For this review, take the finished solid that the model builds, in its own axes (mm). Face numbers are marked on the shaded views. A direction names the side the tool comes from. Give positions to 0.01 mm unless a question says otherwise; leave off trailing zeros. Loops run counter-clockwise (first coordinate to the right, second up) from the corner with the lowest first, then second, coordinate; pieces in that order, holes last. Notation, with made-up numbers: (82.25, 28.5) - (104.25, 28.5) arc R12 ccw to (104.25, 41.5) - close; hole circle Ø2 at (87, -33). An arc over 180 degrees is marked (long way). Answer as CSV lines item,"result".
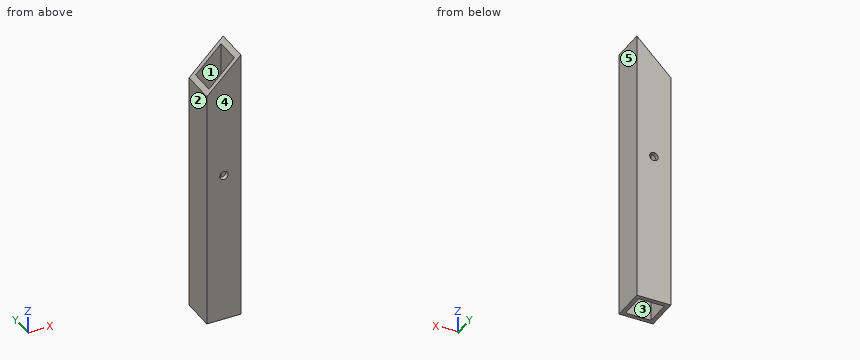
Autodesk Inventor part; units mm, degrees
ref_plane "YZ Plane" through (0, 0, 0) normal (1, 0, 0) x (0, 1, 0)
ref_plane "XZ Plane" through (0, 0, 0) normal (0, 1, 0) x (-1, 0, 0)
ref_plane "XY Plane" through (0, 0, 0) normal (0, 0, 1) x (1, 0, 0)
sketch "Sketch1" plane through (0, 0, 0) normal (0, 0, 1) x (1, 0, 0)
  line L0 (-12.7, 12.7) -> (12.7, 12.7)
  line L1 (12.7, 12.7) -> (12.7, -12.7)
  line L2 (12.7, -12.7) -> (-12.7, -12.7)
  line L3 (-12.7, -12.7) -> (-12.7, 12.7)
  line L4 (-9.525, 9.525) -> (9.525, 9.525)
  line L5 (9.525, 9.525) -> (9.525, -9.525)
  line L6 (9.525, -9.525) -> (-9.525, -9.525)
  line L7 (-9.525, -9.525) -> (-9.525, 9.525)
  point P0 (0, 0)
  dimension "d0" = 25.4
  dimension "d1" = 25.4
  dimension "d2" = 12.7
  dimension "d3" = 12.7
  dimension "d4" = 3.175
  dimension "d5" = 3.175
  dimension "d6" = 3.175
  dimension "d7" = 3.175
extrude "Extrusion1" add sketch "Sketch1" along normal blind 206.375
sketch "Sketch4" plane through (-12.7, 12.7, 0) normal (0, 1, 0) x (1, 0, 0)
  line L0 (0, -206.375) -> (25.4, -206.375)
  line L1 (0, 0) -> (0, -206.375)
  line L2 (25.4, -206.375) -> (0, -180.975)
  point P0 (12.7, 0)
  dimension "d16" = 45
extrude "Extrusion4" cut sketch "Sketch4" against normal blind 25.4
sketch "Sketch5" plane through (-12.7, 12.7, 0) normal (0, 1, 0) x (1, 0, 0)
  line L0 (25.4, 0) -> (25.4, -206.375)
  line L1 (0, 0) -> (25.4, 0)
  circle A0 centre (12.7, -114.3) radius 3.175
  point P0 (12.7, 0)
  dimension "d19" = 114.3
  dimension "d20" = 12.7
  dimension "d21" = 6.35
extrude "Extrusion5" cut sketch "Sketch5" against normal blind 25.4
properties part number "edge frame tube1"
1) Consider section A-A on y = 0. Write out the cut boundary in (x, z) (3 decimals).
From the geometry:
outline,"(-12.7, 0) - (-9.525, 0) - (-9.525, 184.15) - (-12.7, 180.975) - close; (9.525, 0) - (12.7, 0) - (12.7, 206.375) - (9.525, 203.2) - close"
2) Machinability: for the marked faces 1 and 2, which of the approach directions +Z, -Z, +X, -X, +Y, -Y give a long, thin tool a straight path to every point of the face, cutting with its end or side? Answer none if there is none.
From the geometry:
face 1,"+Z, -Z"
face 2,"+Z, -Z, -X, +Y, -Y"
3) Consider section C-C on z = 47. Write out the cut boundary in (x, y) (3 decimals), and give its area (3 significant figures).
From the geometry:
outline,"(-12.7, -12.7) - (12.7, -12.7) - (12.7, 12.7) - (-12.7, 12.7) - close; hole (-9.525, -9.525) - (9.525, -9.525) - (9.525, 9.525) - (-9.525, 9.525) - close"
area,"282 mm^2"
4) Insertion check: P1, Ø5.5, axis at x = 0, z = 114.3, coming from the -Y side. The pin has a flat end and moves straight along its axis. Give the tip position at first contact, or say it passes through.
From the geometry:
P1,"passes through"
5) Consider section B-B on z = 114.3. Write out the cut boundary in (x, y) (3 decimals).
From the geometry:
outline,"(-12.7, -12.7) - (-3.175, -12.7) - (-3.175, -9.525) - (-9.525, -9.525) - (-9.525, 9.525) - (-3.175, 9.525) - (-3.175, 12.7) - (-12.7, 12.7) - close; (3.175, -12.7) - (12.7, -12.7) - (12.7, 12.7) - (3.175, 12.7) - (3.175, 9.525) - (9.525, 9.525) - (9.525, -9.525) - (3.175, -9.525) - close"
6) Consider section D-D on x = 0. Write out the cut boundary in (y, z) (3 decimals), and give its area (3 significant figures).
From the geometry:
outline,"(-12.7, 0) - (-9.525, 0) - (-9.525, 111.125) - (-12.7, 111.125) - close; (-12.7, 117.475) - (-9.525, 117.475) - (-9.525, 193.675) - (-12.7, 193.675) - close; (9.525, 0) - (12.7, 0) - (12.7, 111.125) - (9.525, 111.125) - close; (9.525, 117.475) - (12.7, 117.475) - (12.7, 193.675) - (9.525, 193.675) - close"
area,"1,190 mm^2"
7) Wall thickness on line 1 (X direction, y = -3, z = 33) (3 decimals); line 2 (X direction, y = 11, z = 114.3) (3 decimals): over which ranges is each line inside the solid? List them lowest first. Write a range as from..to.
From the geometry:
line 1,"x = -12.7..-9.525, 9.525..12.7"
line 2,"x = -12.7..-3.175, 3.175..12.7"
8) Draft analysis for pull direction Y (two halves, no side actions). For the marked faces 3, 4 and 5, state which applies: pulls with the +Y half, pulls with the -Y half, needs draft (parallel to the pull), parting line crosses it, or undercut.
From the geometry:
face 3,"undercut"
face 4,"pulls with the -Y half"
face 5,"needs draft"
